Autodesk Inventor part; units mm, degrees
ref_plane "YZ Plane" through (0, 0, 0) normal (1, 0, 0) x (0, 1, 0)
ref_plane "XZ Plane" through (0, 0, 0) normal (0, 1, 0) x (-1, 0, 0)
ref_plane "XY Plane" through (0, 0, 0) normal (0, 0, 1) x (1, 0, 0)
sketch "Эскиз1" plane through (0, 0, 0) normal (0, 1, 0) x (-1, 0, 0)
  circle A0 centre (0, 0) radius 9.5
  dimension "d0" = 19
extrude "Выдавливание1" add sketch "Эскиз1" along normal blind 3.5
sketch "Эскиз2" plane through (0, 3.5, 0) normal (0, 1, 0) x (1, 0, 0)
  circle A0 centre (0, 0) radius 5
  dimension "d3" = 10
extrude "Выдавливание2" add sketch "Эскиз2" along normal blind 8
sketch "Эскиз3" plane through (0, 11.5, 0) normal (0, 1, 0) x (1, 0, 0)
  circle A0 centre (0, 0) radius 9.5
extrude "Выдавливание3" add sketch "Эскиз3" along normal blind 3.5
chamfer "Фаска1" distance 1 angle 45 2 edges at (9.5, 0, 0) (-9.5, 15, 0)
chamfer "Фаска2" distance 0.2 angle 45 2 edges at (-5, 11.5, 0) (-5, 3.5, 0)
sketch "Эскиз4" plane through (0, 15, 0) normal (0, 1, 0) x (1, 0, 0)
  circle A0 centre (0, 0) radius 3.1
  dimension "d14" = 6.2
extrude "Выдавливание4" cut sketch "Эскиз4" against normal through all
properties part number "КВ33.044.402 - Каток" material "ПВХ, непластифицированный"
Input: part model. Units: mm. Frame: model coordinates. A direction names the side the tool comes from. Give positions to 0.01 mm unless a question says otherwise; leave off trailing zeros. Write each loop counter-clockwise with the first axis right and the second up, starting at its lowest first coordinate (ties: lowest second). Pieces come first, ordered by that corner, then holes. Notation, with made-up numbers: (-14, -29) -> (30, -29) arc R24 cw to (30, -5) -> close; hole circle Ø2 at (58.25, 53). An arc over 180 degrees is marked (long way). Use one line per item in the form item = value. Start each with the question number.
1) Pin query (flat end, axial travel): pin 1 (5 mm diameter, centred on y = 13, z = -3.5, fed in from +X); pin 2 (4 mm diameter, centred on y = 6, z = -3.5, fed in from +X); pin 3 (4 mm diameter, centred on y = 3, z = 4.5, fed in from -X); pin 4 (10 mm diameter, centred on x = 0, z = 0, fed in from -Y). Return the tip coordinate at first contact, or that it passes through.
2) Draft query along X for faces 3 (the flat face through (4, 15, 0)), 4 (the cylindrical face through (1.43, 7.6, 2.75)), 5 (the cylindrical face through (-4.38, 2.23, 8.43)). Return one class per face: pulls with the +X half, pulls with the -X half, needs draft (parallel to the pull), parting line crosses it, or undercut.
3) Section query C-C on y = 8.25. Return the cut outline in (x, z).
4) Section query D-D on y = 13.25. Return the cut outline in (x, z), then the cut area to 3 significant figures.
5) Section query A-A on x = 0. Return the cut outline in (y, z).
6) Ray query, probe 1 along X at (y, z) = (10.5, 0); probe 2 along Y at (x, z) = (-7, -1). Return the intervals inside material, ascending. Write a range as from..to.
7) Section query B-B on z = 0. Return the cut outline in (x, y).
8) Set-up query: faces 1 (the cylindrical face through (4.38, 12.73, -8.43)), 2 (the flat face through (-4, 3.5, -4)). Return all of +Z, -Z, +X, -X, +Y, -Y with unobstructed straight access to the full face (end or side cutting, diameter ignored); none if empty.
Outcome:
q1.pin_1 = 9.45
q1.pin_2 = 4.77
q1.pin_3 = -9.17
q1.pin_4 = 0
q2.face_3 = needs draft
q2.face_4 = undercut
q2.face_5 = parting line crosses it
q3.outline = circle Ø10 at (0, 0); hole circle Ø6.2 at (0, 0)
q4.outline = circle Ø19 at (0, 0); hole circle Ø6.2 at (0, 0)
q4.area = 253 mm^2
q5.outline = (0, -8.5) -> (1, -9.5) -> (3.5, -9.5) -> (3.5, -5.2) -> (3.7, -5) -> (11.3, -5) -> (11.5, -5.2) -> (11.5, -9.5) -> (14, -9.5) -> (15, -8.5) -> (15, -3.1) -> (0, -3.1) -> close; (0, 3.1) -> (15, 3.1) -> (15, 8.5) -> (14, 9.5) -> (11.5, 9.5) -> (11.5, 5.2) -> (11.3, 5) -> (3.7, 5) -> (3.5, 5.2) -> (3.5, 9.5) -> (1, 9.5) -> (0, 8.5) -> close
q6.probe_1 = -5..-3.1, 3.1..5
q6.probe_2 = 0..3.5, 11.5..15
q7.outline = (-9.5, 1) -> (-8.5, 0) -> (-3.1, 0) -> (-3.1, 15) -> (-8.5, 15) -> (-9.5, 14) -> (-9.5, 11.5) -> (-5.2, 11.5) -> (-5, 11.3) -> (-5, 3.7) -> (-5.2, 3.5) -> (-9.5, 3.5) -> close; (3.1, 0) -> (8.5, 0) -> (9.5, 1) -> (9.5, 3.5) -> (5.2, 3.5) -> (5, 3.7) -> (5, 11.3) -> (5.2, 11.5) -> (9.5, 11.5) -> (9.5, 14) -> (8.5, 15) -> (3.1, 15) -> close
q8.face_1 = +Y, -Y
q8.face_2 = none
